Autodesk Inventor part; units mm, degrees
ref_plane "Start Plane" through (0, 0, 0) normal (0, 0, 1) x (1, 0, 0)
ref_plane "End Plane" through (0, 0, 60.325) normal (0, 0, 1) x (1, 0, 0)
ref_plane "Work Plane5" through (-25.4, 419.1, 60.325) normal (0, 0, 1) x (1, 0, 0)
ref_plane "Start Plane" through (0, 0, 0) normal (0, 0, 1) x (1, 0, 0)
ref_plane "End Plane" through (0, 0, 60.325) normal (0, 0, 1) x (1, 0, 0)
sketch "Sketch" plane through (0, 0, 0) normal (0, 0, 1) x (1, 0, 0)
  line L0 (-25.4, -12.7) -> (25.4, -12.7)
  line L1 (25.4, -12.7) -> (25.4, 12.7)
  line L2 (25.4, 12.7) -> (-25.4, 12.7)
  line L3 (-25.4, 12.7) -> (-25.4, -12.7)
  line L4 (-25.4, -12.7) -> (25.4, 12.7) construction
  line L5 (25.4, -12.7) -> (-25.4, 12.7) construction
  line L6 (-22.225, -9.525) -> (22.225, -9.525)
  line L7 (22.225, -9.525) -> (22.225, 9.525)
  line L8 (22.225, 9.525) -> (-22.225, 9.525)
  line L9 (-22.225, 9.525) -> (-22.225, -9.525)
  line L10 (-22.225, -9.525) -> (22.225, 9.525) construction
  line L11 (22.225, -9.525) -> (-22.225, 9.525) construction
  point P0 (0, 0)
  point P1 (0, 0)
  dimension "d0" = 50.8
  dimension "d1" = 25.4
  dimension "d2" = 3.175
  dimension "d3" = 3.175
extrude "Body" add sketch "Sketch" along normal up to surface (60.325 mm away) from surface at 0
sketch "Sketch4" plane through (0, 0, 0) normal (0, 0, 1) x (1, 0, 0)
  line L0 (0, 0) -> (10, 0)
ref_plane "Work Plane4" through (0, 0, 0) normal (0, -1, 0) x (1, 0, 0)
sketch "Sketch5" plane through (0, 0, 0) normal (0, -1, 0) x (1, 0, 0)
  line L0 (-2, 0) -> (12, 0)
  line L1 (-2, 60.325) -> (12, 60.325)
  dimension "d11" = 60.325
ref_plane "Work Plane5" through (-25.4, 419.1, 60.325) normal (0, 0, 1) x (1, 0, 0)
split "Split1" plane through (-25.4, 419.1, 60.325) removes the side toward (0, 0, 1)
equation "\"G_OFFSET_START\" = 0"
equation "\"G_OFFSET_END\" = -12.7"
equation "\"d7\" = length + G_OFFSET_END"
equation "\"G_L\" = d11"
properties part number "2x1inTubing"
The listing builds one solid part. Answer for the finished solid, in the listing's coordinates (mm). A direction names the side the tool comes from. Give positions to 0.01 mm unless a question says otherwise; leave off trailing zeros. Loops run counter-clockwise (first coordinate to the right, second up) from the corner with the lowest first, then second, coordinate; pieces in that order, holes last.
Item 1: Find the intervals of material crossed by line 1 along X through (y, z) = (1.75, 46) (3 decimals); line 2 along Y through (x, z) = (-5, 17) (3 decimals), in increasing order.
Derived:
line 1: x = -25.4 to -22.225, 22.225 to 25.4
line 2: y = -12.7 to -9.525, 9.525 to 12.7
Item 2: A tool of negligible diameter and unlimited length cuts with its end or side. For faces 1 (the flat face through (0, 12.7, 30)), 2 (the flat face through (22.225, 0, 30)), from which of +Z, -Z, +X, -X, +Y, -Y can it reach the whole face along a straight path? Write none if from no direction.
Derived:
face 1: +Z, -Z, +X, -X, +Y
face 2: +Z, -Z
Item 3: A cutting plane is placed at C-C (z = 7.5). Give the vertices of the cut face in (x, y) (3 decimals).
Derived:
outline: (-25.4, -12.7) - (25.4, -12.7) - (25.4, 12.7) - (-25.4, 12.7) - close; hole (-22.225, -9.525) - (22.225, -9.525) - (22.225, 9.525) - (-22.225, 9.525) - close
Item 4: Determine the mould class of faces 3 (the flat face through (0, -12.7, 30)), 4 (the flat face through (0, -9.525, 30)), 5 (the flat face through (0, 9.525, 30)), 6 (the flat face through (-25.4, 0, 30)) for opening direction Y: +Y half, -Y half, draft (parallel to the pull), parting line (faces both ways), or undercut.
Derived:
face 3: -Y half
face 4: undercut
face 5: undercut
face 6: draft
Item 5: A cutting plane is placed at A-A (y = 8). Give the vertices of the cut face in (x, z) (3 decimals).
Derived:
outline: (-25.4, 0) - (-22.225, 0) - (-22.225, 60.325) - (-25.4, 60.325) - close; (22.225, 0) - (25.4, 0) - (25.4, 60.325) - (22.225, 60.325) - close
Item 6: A cutting plane is placed at B-B (x = -14.5). Give the vertices of the cut face in (y, z) (3 decimals), then the cut area to 3 significant figures.
Derived:
outline: (-12.7, 0) - (-9.525, 0) - (-9.525, 60.325) - (-12.7, 60.325) - close; (9.525, 0) - (12.7, 0) - (12.7, 60.325) - (9.525, 60.325) - close
area: 383 mm2
